Verification items for the finished model (mm, model axes). Face numbers are marked on the shaded views. Round coordinates to 2 decimals unless told otherwise and drop trailing zeros. Order: outer loops, then holes, each group sorted by start corner. A loop starts at its lowest first (then second) coordinate and runs counter-clockwise, first axis right, second up. Notation, with made-up numbers: M 86.5,72 L 102.5,72 A24 cw 102.5,95 Z; hole C -29.75,87.5 d11. An arc over 180 degrees is marked long. Return JSON: item names as keys, results as strings. Group by question number.
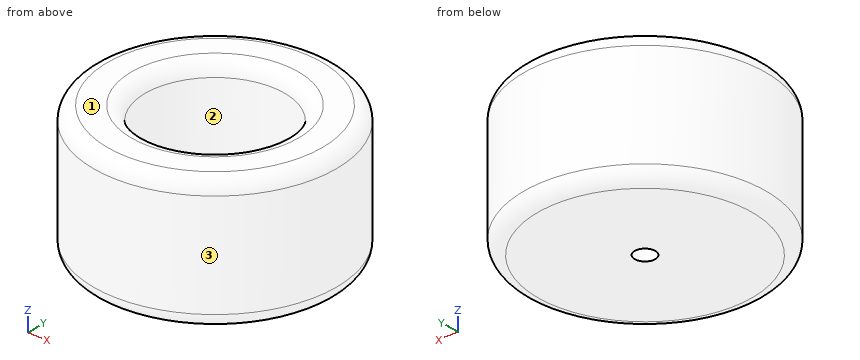
Autodesk Inventor part; units mm, degrees
ref_plane "YZ Plane" through (0, 0, 0) normal (1, 0, 0) x (0, 1, 0)
ref_plane "XZ Plane" through (0, 0, 0) normal (0, 1, 0) x (-1, 0, 0)
ref_plane "XY Plane" through (0, 0, 0) normal (0, 0, 1) x (1, 0, 0)
sketch "Sketch1" plane through (0, 0, 0) normal (0, 0, 1) x (1, 0, 0)
  circle A0 centre (0, 0) radius 10.05
  circle A1 centre (0, 0) radius 17.5
  dimension "d0" = 20.1
  dimension "d2" = 35
extrude "Extrusion1" add sketch "Sketch1" against normal blind 19
sketch "Sketch2" plane through (0, 0, -19) normal (0, 0, -1) x (-1, 0, 0)
  circle A0 centre (0, 0) radius 10.05
  circle A1 centre (0, 0) radius 1.5
  dimension "d7" = 3
extrude "Extrusion2" add sketch "Sketch2" against normal blind 3.5 contours A0 | A1
extrude "Extrusion3" cut sketch "Sketch2" against normal blind 3.5 contours A1
fillet "Fillet1" radius 2 1 edges at (-10.05, 0, 0)
fillet "Fillet2" radius 2 2 edges at (-17.5, 0, 0) (-17.5, 0, -19)
properties part number "rulmanyatagıipt"
1. Draft check along Y on the marked faces 1, 2 and 3. Enter one of: +Y half, -Y half, draft (parallel to the pull), parting line (faces both ways), or undercut.
2. Cross-section at C-C (z = -16.5). Enter the section's corners in (x, y), plus the area to 3 significant figures.
3. Cross-section at D-D (z = -11). Enter the section's corners in (x, y), plus the area to 3 significant figures.
4. Thickness scan on line 1 along Y through (x, z) = (0, -17.1); line 2 along Y through (x, z) = (-8, -13); line 3 along X through (y, z) = (-7.5, -13.75). Record the ranges inside material, lowest first. Write a range as from..to.
5. Cross-section at A-A (y = 0). Enter the section's corners in (x, z), plus the area to 3 significant figures.
6. Go/stop test with flat-tipped pins: pin 1 (8 mm diameter, centred on x = 11.5, y = -11, fed in from -Z); pin 2 (1.5 mm diameter, centred on x = -10, z = -9.5, fed in from +Y); pin 3 (8 mm diameter, centred on x = -12, z = -15.5, fed in from -Y); pin 4 (1.5 mm diameter, centred on y = 4.5, z = -12.5, fed in from +X). Record where each tip stops, or that it passes through.
Computed:
{
 "1": {"face 1": "draft", "face 2": "undercut", "face 3": "parting line"},
 "2": {"outline": "C 0,0 d35; hole C 0,0 d3", "area": "955 mm²"},
 "3": {"outline": "C 0,0 d35; hole C 0,0 d20.1", "area": "645 mm²"},
 "4": {"line 1": "y = -17.5..-1.5, 1.5..17.5", "line 2": "y = -15.56..-6.08, 6.08..15.56", "line 3": "x = -15.81..-6.69, 6.69..15.81"},
 "5": {"outline": "M -17.5,-17 A2 ccw -15.5,-19 L -1.5,-19 L -1.5,-15.5 L -10.05,-15.5 L -10.05,-2 A2 ccw -12.05,0 L -15.5,0 A2 ccw -17.5,-2 Z; M 1.5,-19 L 15.5,-19 A2 ccw 17.5,-17 L 17.5,-2 A2 ccw 15.5,0 L 12.05,0 A2 ccw 10.05,-2 L 10.05,-15.5 L 1.5,-15.5 Z", "area": "338 mm²"},
 "6": {"pin 1": "stops at z = -19", "pin 2": "stops at y = 14.86", "pin 3": "stops at y = -15.56", "pin 4": "stops at x = 17.09"}
}
